```python
from build123d import *

# Parameters (mm, degrees)
EXTRUDE_1_DEPTH          = 5
SKETCH_2_R               = 4
CUT_EXTRUDE_1_DEPTH      = 6
PATTERN_CIRCULAR_1_COUNT = 3
SKETCH_3_R               = 4
CUT_EXTRUDE_2_DEPTH      = 6
PATTERN_CIRCULAR_2_COUNT = 3
SKETCH_4_R               = 4
CUT_EXTRUDE_3_DEPTH      = 6
PATTERN_CIRCULAR_3_COUNT = 3
FILLET_1_R               = 50


with BuildPart() as part:
    # Sketch 1 → Extrude 1 (new body)
    with BuildSketch(Plane(origin=(0, 0, 0), x_dir=(1, 0, 0), z_dir=(0, 1, 0))):
        Polygon((57.735026919, 100), (-57.735026919, 100), (-115.470053838, 0), (-57.735026919, -100), (57.735026919, -100), (115.470053838, 0), align=None)
    extrude(amount=EXTRUDE_1_DEPTH)

    # Sketch 2 → Cut-Extrude 1 (cut, through all)
    with BuildSketch(Plane(origin=(0, 5, 0), x_dir=(1, 0, 0), z_dir=(0, 1, 0))):
        with Locations((-23.5, 37)):
            Circle(SKETCH_2_R)
        with Locations((23.5, 37)):
            Circle(SKETCH_2_R)
        with Locations((-23.5, 63)):
            Circle(SKETCH_2_R)
        with Locations((23.5, 63)):
            Circle(SKETCH_2_R)
        with Locations((-23.5, 89)):
            Circle(SKETCH_2_R)
        with Locations((23.5, 89)):
            Circle(SKETCH_2_R)
    cut_extrude_1 = extrude(amount=-CUT_EXTRUDE_1_DEPTH, mode=Mode.SUBTRACT)

    # Pattern Circular 1: Cut-Extrude 1 ×3 about axis
    pattern_circular_1_axis = Axis((0, 0, 0), (0, 1, 0))
    for i in range(1, PATTERN_CIRCULAR_1_COUNT):
        add(cut_extrude_1.rotate(pattern_circular_1_axis, i * 360 / PATTERN_CIRCULAR_1_COUNT), mode=Mode.SUBTRACT)

    # Sketch 3 → Cut-Extrude 2 (cut, through all)
    with BuildSketch(Plane(origin=(0, 5, 0), x_dir=(1, 0, 0), z_dir=(0, 1, 0))):
        with Locations((65.326260937, 64.851596989)):
            Circle(SKETCH_3_R)
        with Locations((88.826260937, 24.148403011)):
            Circle(SKETCH_3_R)
        with Locations((54.559600438, 31.5)):
            Circle(SKETCH_3_R)
    cut_extrude_2 = extrude(amount=-CUT_EXTRUDE_2_DEPTH, mode=Mode.SUBTRACT)

    # Pattern Circular 2: Cut-Extrude 2 ×3 about axis
    pattern_circular_2_axis = Axis((0, 0, 0), (0, 1, 0))
    for i in range(1, PATTERN_CIRCULAR_2_COUNT):
        add(cut_extrude_2.rotate(pattern_circular_2_axis, i * 360 / PATTERN_CIRCULAR_2_COUNT), mode=Mode.SUBTRACT)

    # Sketch 4 → Cut-Extrude 3 (cut, through all)
    with BuildSketch(Plane(origin=(0, 5, 0), x_dir=(1, 0, 0), z_dir=(0, 1, 0))):
        with Locations((0, 20)):
            Circle(SKETCH_4_R)
    cut_extrude_3 = extrude(amount=-CUT_EXTRUDE_3_DEPTH, mode=Mode.SUBTRACT)

    # Pattern Circular 3: Cut-Extrude 3 ×3 about axis
    pattern_circular_3_axis = Axis((0, 0, 0), (0, 1, 0))
    for i in range(1, PATTERN_CIRCULAR_3_COUNT):
        add(cut_extrude_3.rotate(pattern_circular_3_axis, i * 360 / PATTERN_CIRCULAR_3_COUNT), mode=Mode.SUBTRACT)

    # Fillet 1
    fillet_1_edges = [part.edges().sort_by_distance(p)[0] for p in [
        (115.470053838, 2.5, 0),
        (57.735026919, 2.5, 100),
        (-57.735026919, 2.5, 100),
        (-115.470053838, 2.5, 0),
        (-57.735026919, 2.5, -100),
        (57.735026919, 2.5, -100),
    ]]
    fillet(fillet_1_edges, radius=FILLET_1_R)


solid = part.part
```
For this review, take the finished solid that the model builds, in its own axes (mm). Round coordinates to 2 decimals unless told otherwise and drop trailing zeros. Write each loop counter-clockwise with the first axis right and the second up, starting at its lowest first coordinate (ties: lowest second). Pieces come first, ordered by that corner, then holes. Notation, with made-up numbers: (-1, -5.5) - (52, -5.5) arc R23 ccw to (52, 16.5) - close; hole circle Ø2 at (43.25, -24.75). An arc over 180 degrees is marked (long way). Answer as a JSON object with one key per item and string values.
1. We need section C-C on x = 77. Give the boundary of the cut face in (y, z), then the cut area to 3 significant figures.
Response values:
{"outline": "(0, -66.63) - (5, -66.63) - (5, 66.63) - (0, 66.63) - close", "area": "666 mm2"}
2. Draft analysis for pull direction Z (two halves, no side actions). For faces 1 (the face through (-107.734, 2.535, -0.367)), 2 (the face through (62.152, 2.535, 67.286)), 3 (the face through (53.549, 2.535, -93.483)), state which applies: +Z half, -Z half, draft (parallel to the pull), parting line (faces both ways), or undercut.
Response values:
{"face 1": "parting line", "face 2": "undercut", "face 3": "-Z half"}
3. For pin 1 Ø2 at (y, z) = (0.5, 38) entering from -X; pin 2 Ø2 at (y, z) = (1.5, -54.5) entering from +X, all flat-tipped, find the tip position at first contact; note any pin that passes through.
Response values:
{"pin 1": "stops at x = -94.11", "pin 2": "stops at x = 84.58"}
4. We need section B-B on y = 2.4. Count the separate pieces of the cut face and the enclosed holes in it, then the cut area to 3 significant figures.
Response values:
{"separate pieces": "1", "enclosed holes": "30", "area": "32,300 mm2"}
5. We need section A-A on z = -89. Give the boundary of the cut face in (x, y).
Response values:
{"outline": "(-60.16, 0) - (-27.5, 0) - (-27.5, 5) - (-60.16, 5) - close; (-19.5, 0) - (19.5, 0) - (19.5, 5) - (-19.5, 5) - close; (27.5, 0) - (60.16, 0) - (60.16, 5) - (27.5, 5) - close"}
6. To check wall thickness, follow line 1 along Z through (x, y) = (-42, 3.7); line 2 along X through (y, z) = (4.15, -85.5); line 3 along X through (y, z) = (3.3, 67.5). State the ranges of each line that lie inside material, in increasing order.
Response values:
{"line 1": "z = -98.24 to -5.43, 1.72 to 47.93, 55.77 to 98.24", "line 2": "x = -64.08 to -25.44, -21.56 to 21.56, 25.44 to 64.08", "line 3": "x = -76.5 to -68.32, -62.33 to 62.33, 68.32 to 76.5"}
